Part model, mm, in its own coordinate system. A direction names the side the tool comes from. Give positions to 0.01 mm unless a question says otherwise; leave off trailing zeros. Return JSON: item names as keys, results as strings.
from build123d import *

# Parameters (mm, degrees)
F2_R     = 25
F3_DEPTH = 55.001


with BuildPart() as f1:
    # F0 (on Right) → F1 (revolve)
    with BuildSketch(Plane.YZ):
        Polygon((0, 92), (0, 0), (55, 0), (55, 92), (49.063487, 92), (45.713487, 83), (43.713487, 83), (40.363487, 92), (37.587829, 92), (34.237829, 83), (32.237829, 83), (28.887829, 92), (26.112171, 92), (22.762171, 83), (20.762171, 83), (17.412171, 92), (14.636513, 92), (11.286513, 83), (9.286513, 83), (5.936513, 92), align=None)
    revolve(axis=Axis((0, 27.5, 0), (0, 1, 0)))

    # F2 (on face) → F3 (cut, through all)
    with BuildSketch(Plane.XZ):
        Circle(F2_R)
    extrude(amount=-F3_DEPTH, mode=Mode.SUBTRACT)


solid = f1.part
Q1. Probe line 1 along Y through (x, z) = (-82.5, -31); line 2 along Z through (x, y) = (-26.5, 11); line 3 along X through (y, z) = (34, -5). List the from-to ranges inside material, lowest first.
Established:
{"line 1": "y = 0 to 7.38, 13.2 to 18.85, 24.67 to 30.33, 36.15 to 41.8, 47.62 to 55", "line 2": "z = -78.66 to 78.66", "line 3": "x = -82.85 to -24.49, 24.49 to 82.85"}
Q2. Pin check, flat tips, straight feed: pin 1 (8 mm diameter, centred on y = 47, z = -40.5, fed in from -X); pin 2 (5 mm diameter, centred on y = 16, z = -71.5, fed in from +X). Stop position of each tip, or through.
Established:
{"pin 1": "stops at x = -84.2", "pin 2": "stops at x = 60.85"}
Q3. Two-plate mould, pull along Y, no slides. Class faces 3 (the flat face through (-19, 55, -19)), 4 (the conical face through (-81.576, 32.028, -18.115)), 5 (the cylindrical face through (91.217, 38.956, -11.977)): +Y half, -Y half, draft (parallel to the pull), parting line (faces both ways), or undercut.
Established:
{"face 3": "+Y half", "face 4": "undercut", "face 5": "draft"}
Q4. 3-axis set-ups, long thin cutter, end or side, ignore diameter. For faces 1 (the conical face through (-81.58, 20.55, -18.11)), 2 (the cylindrical face through (91.217, 27.481, -11.977)): which of +Z, -Z, +X, -X, +Y, -Y reach the whole face in a straight line?
Established:
{"face 1": "none", "face 2": "+Y, -Y"}
